Check sheet for the drawn part. Datum: minimum x, y, z corner. Units: mm. A direction names the side the tool comes from. Give positions to 0.01 mm unless a question says otherwise; leave off trailing zeros. Order: outer loops, then holes, each group sorted by start corner. A loop starts at its lowest first (then second) coordinate and runs counter-clockwise, first axis right, second up. Notation, with made-up numbers: (22, -29.75) -> (52, -29.75) arc R27 ccw to (52, -12.75) -> close; hole circle Ø8 at (57.25, 75.25). An arc over 180 degrees is marked (long way). Return JSON: item names as keys, results as strings. Group by question number.
(1) Cross-section at A-A on z = 4. Enter the section's corners in (x, y).
(2) Thickness scan on line 1 along Z through (x, y) = (4, 6); line 2 along Y through (x, z) = (5.5, 6.75); line 3 along X through (y, z) = (20.5, 5.25). Record the ranges inside material, lowest first.
(3) Cross-section at D-D on y = 30.5. Enter the section's corners in (x, z).
(4) Cross-section at B-B on x = 4. Enter the section's corners in (y, z), then the cut area to 3 significant figures.
(5) Depth check by flat-ended pin: pin 1 Ø3 at (y, z) = (21.5, 1) entering from +X. Enter the tip coordinate at first touch or a pass-through.
(6) Tool access check on the marked faces 1 and 2. Record the directions out of +Z, -Z, +X, -X, +Y, -Y that give a thin tool (end or side, any length) a straight path to the whole face; none if there is none.
(7) Cross-section at C-C on y = 9. Enter the section's corners in (x, z).
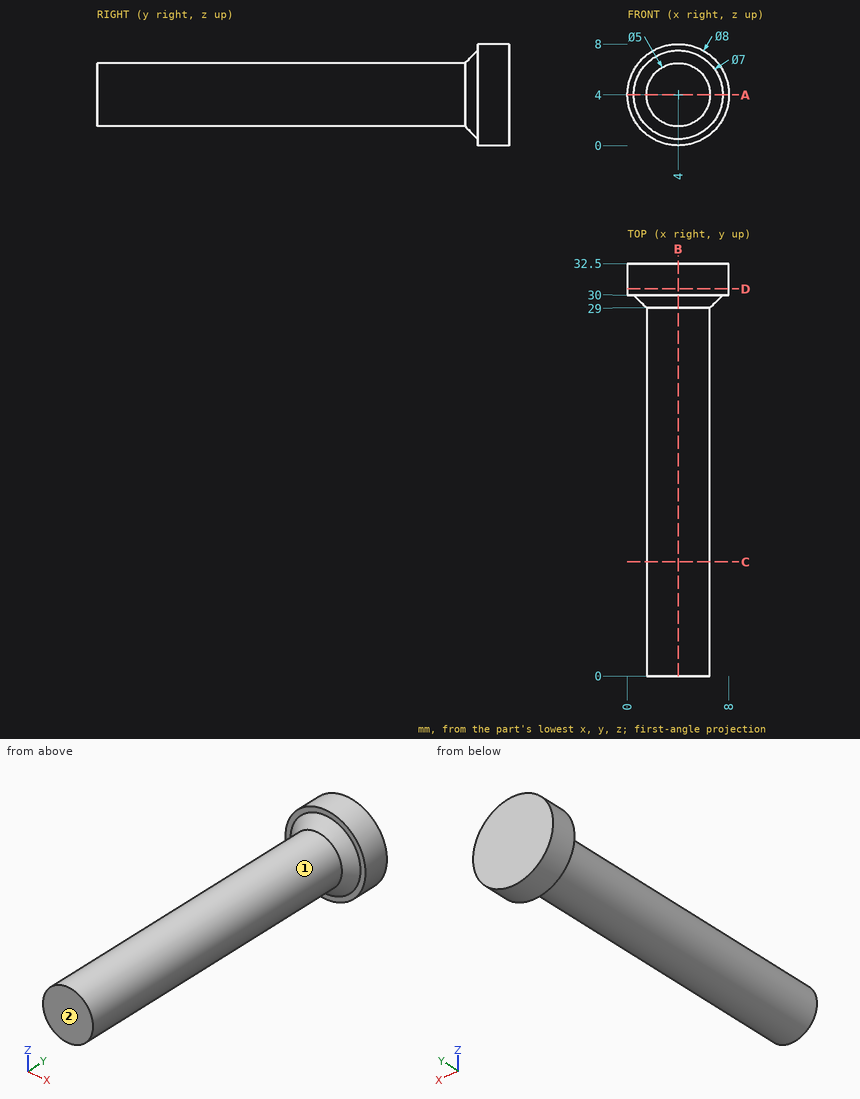
Verdict:
{
 "1": {"outline": "(0, 30) -> (0.5, 30) -> (1.5, 29) -> (1.5, 0) -> (6.5, 0) -> (6.5, 29) -> (7.5, 30) -> (8, 30) -> (8, 32.5) -> (0, 32.5) -> close"},
 "2": {"line 1": "1.5 to 6.5", "line 2": "29.63 to 32.5", "line 3": "1.83 to 6.17"},
 "3": {"outline": "circle Ø8 at (4, 4)"},
 "4": {"outline": "(0, 1.5) -> (29, 1.5) -> (30, 0.5) -> (30, 0) -> (32.5, 0) -> (32.5, 8) -> (30, 8) -> (30, 7.5) -> (29, 6.5) -> (0, 6.5) -> close", "area": "171 mm²"},
 "5": {"pin 1": "x = 6"},
 "6": {"face 1": "-Y", "face 2": "+Z, -Z, +X, -X, -Y"},
 "7": {"outline": "circle Ø5 at (4, 4)"}
}
